from build123d import *

# Parameters (mm, degrees)
SKETCH1_W           = 71.12
SKETCH1_H           = 71.12
BOSS_EXTRUDE1_DEPTH = 4.7625
SKETCH2_R           = 3.4925
CUT_EXTRUDE1_DEPTH  = 51.514439582
SKETCH3_R           = 12.425
BOSS_EXTRUDE2_DEPTH = 49
SKETCH5_R           = 1.27
BOSS_EXTRUDE3_DEPTH = 10
FILLET1_R           = 2.5
SKETCH6_W           = 86.163151286
SKETCH6_H           = 93.634187614
CUT_EXTRUDE2_DEPTH  = 4.7625
SKETCH7_R           = 2.667
CUT_EXTRUDE3_DEPTH  = 10


with BuildPart() as part:
    # Sketch1 → Boss-Extrude1 (new body)
    with BuildSketch(Plane.XY):
        Rectangle(SKETCH1_W, SKETCH1_H)
    extrude(amount=BOSS_EXTRUDE1_DEPTH)

    # Sketch2 → Cut-Extrude1 (cut, through all)
    with BuildSketch(Plane.XY.offset(4.7625)):
        with Locations((-30.48, 30.48)):
            Circle(SKETCH2_R)
        with Locations((30.48, 30.48)):
            Circle(SKETCH2_R)
    cut_extrude1 = extrude(amount=-CUT_EXTRUDE1_DEPTH, mode=Mode.SUBTRACT)

    # Mirror1: Cut-Extrude1 across plane
    add(cut_extrude1.mirror(Plane.ZX), mode=Mode.SUBTRACT)

    # Sketch3 → Boss-Extrude2 (add)
    with BuildSketch(Plane.XY.offset(4.7625)):
        Circle(SKETCH3_R)
    extrude(amount=BOSS_EXTRUDE2_DEPTH)

    # Sketch4 → Cut-Revolve1 (revolve, cut)
    with BuildSketch(Plane(origin=(0, 0, 0), x_dir=(0, 0, -1), z_dir=(1, 0, 0)), mode=Mode.PRIVATE) as cut_revolve1_sk:
        Polygon((-4.7625, 12.425), (-53.7625, 1.245), (-53.7625, 12.425), align=None)
    revolve(cut_revolve1_sk.sketch.rotate(Axis((0, 0, 53.7625), (0, 0, -1)), 270), axis=Axis((0, 0, 53.7625), (0, 0, -1)), mode=Mode.SUBTRACT)

    # Sketch5 → Boss-Extrude3 (add)
    with BuildSketch(Plane.XY.offset(53.7625)):
        Circle(SKETCH5_R)
    extrude(amount=BOSS_EXTRUDE3_DEPTH)

    # Fillet1
    fillet1_edges = [part.edges().sort_by_distance(p)[0] for p in [
        (-35.56, 35.56, 2.38125),
        (35.56, 35.56, 2.38125),
        (35.56, -35.56, 2.38125),
        (-35.56, -35.56, 2.38125),
    ]]
    fillet(fillet1_edges, radius=FILLET1_R)

    # Sketch6 → Cut-Extrude2 (cut)
    with BuildSketch(Plane(origin=(0, 0, 0), x_dir=(-1, 0, 0), z_dir=(0, 0, -1))):
        Rectangle(SKETCH6_W, SKETCH6_H)
    extrude(amount=-CUT_EXTRUDE2_DEPTH, mode=Mode.SUBTRACT)

    # Sketch7 → Cut-Extrude3 (cut)
    with BuildSketch(Plane(origin=(0, 0, 4.7625), x_dir=(-1, 0, 0), z_dir=(0, 0, -1))):
        Circle(SKETCH7_R)
    extrude(amount=-CUT_EXTRUDE3_DEPTH, mode=Mode.SUBTRACT)


solid = part.part
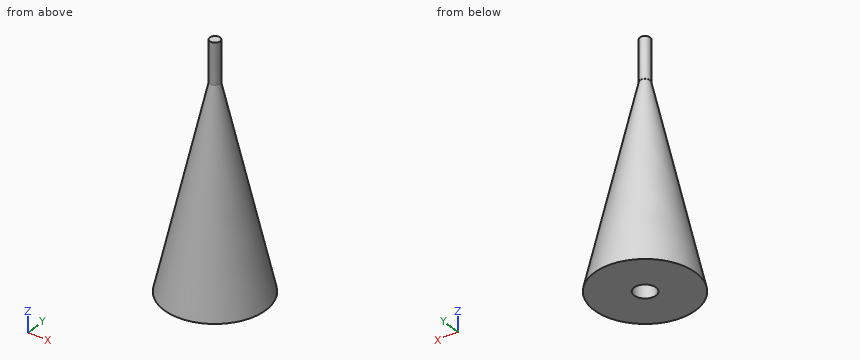
Geometry: final body of the model. Coordinates: model frame, mm. Round coordinates to 2 decimals unless told otherwise and drop trailing zeros. Loops run counter-clockwise (first coordinate to the right, second up) from the corner with the lowest first, then second, coordinate; pieces in that order, holes last. Notation, with made-up numbers: M 3,71 L 37,71 A18 cw 37,106 Z; hole C -37,48 d5. An arc over 180 degrees is marked long. One line per question, with ' | ' between items.
(1) Material intervals for line 1 along Y through (x, z) = (0, 7); line 2 along Y through (x, z) = (0, 11.5); line 3 along Y through (x, z) = (8.5, 18.5), sorted ascending. Write a range as from..to.
Check result:
line 1: y = -11.91..-2.67, 2.67..11.91 | line 2: y = -10.89..-2.67, 2.67..10.89 | line 3: y = -3.75..3.75
(2) Cut plane C-C on z = 15.5. Return the cut outline in (x, y).
Check result:
outline: C 0,0 d19.95
(3) Contact query for flat-ended pins moving along their axis: P1, Ø5, axis at x = -8, z = 11.5, coming from the -Y side; P2, Ø0.8, axis at x = 0, y = 0.5, coming from the -Z side; P3, Ø6, axis at y = -3, z = 38.5, coming from the +X side. Output: stop coordinate, or through.
Check result:
P1: stops at y = -9.54 | P2: stops at z = 14.76 | P3: stops at x = 5.14
(4) Cut plane D-D on z = 45. Return the cut outline in (x, y), plus the area to 3 significant figures.
Check result:
outline: C 0,0 d6.49 | area: 33.1 mm2
